Source: three-view drawing plus pictorial views. Frame: mm from the lowest corner of the part. A direction names the side the tool comes from. Give positions to 0.01 mm unless a question says otherwise; leave off trailing zeros. Order: outer loops, then holes, each group sorted by start corner. A loop starts at its lowest first (then second) coordinate and runs counter-clockwise, first axis right, second up. Notation, with made-up numbers: (71.5, 43) - (105.5, 43) arc R22 ccw to (105.5, 81) - close; hole circle Ø6 at (2, 78.25). An arc over 180 degrees is marked (long way). Answer in a Markdown table with one row per item. Add a question column.
1. Section query C-C on x = 9.5. Return loops of the section in (y, z), and give its area (3 significant figures).
2. Mould query, pull axis X, two halves, no side actions, for the marked faces 1, 2, 3 and 4. Classes: released by +X, released by -X, zero draft, split by the parting line, or undercut.
3. Ray query, line 1 (X direction, y = 10.5, z = 9.4); line 2 (Y direction, x = 8.25, z = 7); line 3 (Y direction, x = 11.5, z = 9.75). Return the intervals inside material, ascending. Write a range as [from, to].
4. Section query D-D on x = 11.5. Return loops of the section in (y, z).
5. Section query B-B on y = 10.5. Return loops of the section in (x, z), and give its area (3 significant figures).
6. Section query A-A on z = 3. Return loops of the section in (x, y).
7. Access query for the marked faces 5, 6 and 7. Directions: +Z, -Z, +X, -X, +Y, -Y. A direction counts if a zero-diameter tool reaches every point of the face in a straight line with its end or side. Return the directions, or none.
8. Contact query for flat-ended pins moving along their axis: pin 1 (6 mm diameter, centred on y = 12, z = 5, fed in from -X); pin 2 (2 mm diameter, centred on x = 15, y = 2, fed in from +Z); pin 3 (8 mm diameter, centred on x = 17, y = 11, fed in from -Z); pin 4 (5 mm diameter, centred on x = 5.5, z = 8.5, fed in from +Y). Output: stop coordinate, or through.
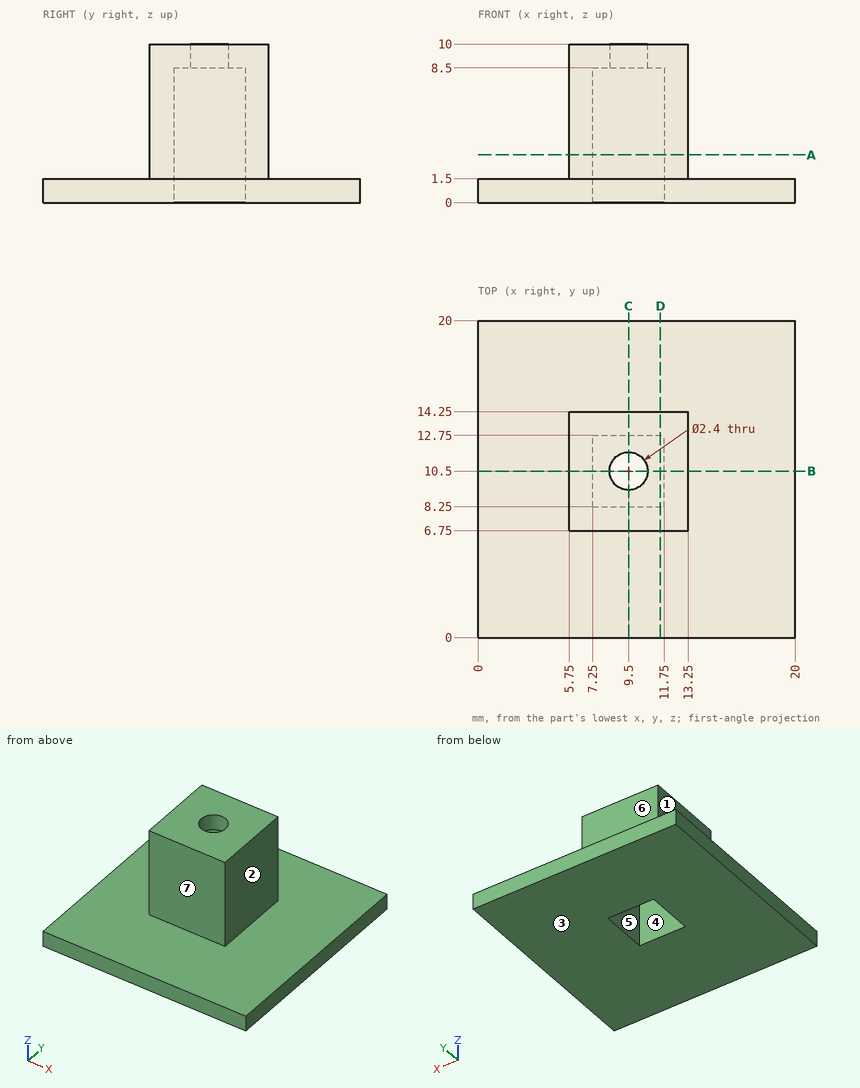
Answer:
| question | item | result |
|---|---|---|
| 1 | outline | (0, 0) - (8.25, 0) - (8.25, 8.5) - (9.3, 8.5) - (9.3, 10) - (6.75, 10) - (6.75, 1.5) - (0, 1.5) - close; (11.7, 8.5) - (12.75, 8.5) - (12.75, 0) - (20, 0) - (20, 1.5) - (14.25, 1.5) - (14.25, 10) - (11.7, 10) - close |
| 1 | area | 51.9 mm² |
| 2 | face 1 | released by -X |
| 2 | face 2 | released by +X |
| 2 | face 3 | zero draft |
| 2 | face 4 | undercut |
| 3 | line 1 | x = [5.75, 8.3], [10.7, 13.25] |
| 3 | line 2 | y = [6.75, 8.25], [12.75, 14.25] |
| 3 | line 3 | y = [6.75, 14.25] |
| 4 | outline | (0, 0) - (8.25, 0) - (8.25, 8.5) - (12.75, 8.5) - (12.75, 0) - (20, 0) - (20, 1.5) - (14.25, 1.5) - (14.25, 10) - (6.75, 10) - (6.75, 1.5) - (0, 1.5) - close |
| 5 | outline | (0, 0) - (7.25, 0) - (7.25, 8.5) - (8.3, 8.5) - (8.3, 10) - (5.75, 10) - (5.75, 1.5) - (0, 1.5) - close; (10.7, 8.5) - (11.75, 8.5) - (11.75, 0) - (20, 0) - (20, 1.5) - (13.25, 1.5) - (13.25, 10) - (10.7, 10) - close |
| 5 | area | 51.9 mm² |
| 6 | outline | (5.75, 6.75) - (13.25, 6.75) - (13.25, 14.25) - (5.75, 14.25) - close; hole (7.25, 8.25) - (11.75, 8.25) - (11.75, 12.75) - (7.25, 12.75) - close |
| 7 | face 5 | -Z |
| 7 | face 6 | +Z, +X, -X, +Y |
| 7 | face 7 | +Z, +X, -X, -Y |
| 8 | pin 1 | stops at x = 5.75 |
| 8 | pin 2 | stops at z = 1.5 |
| 8 | pin 3 | stops at z = 0 |
| 8 | pin 4 | stops at y = 14.25 |
